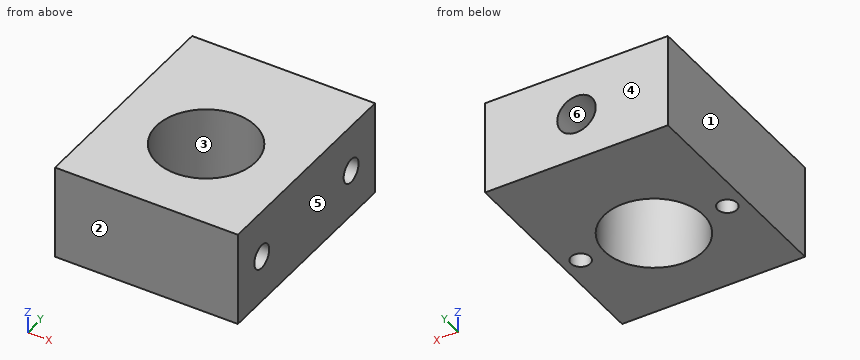
from build123d import *

# Parameters (mm, degrees)
F0_W     = 19
F0_H     = 23
F0_R     = 5.15
F1_DEPTH = 9.8
F3_D     = 2
F3_DEPTH = 5
F3_TIP   = 0.600860619
F5_D     = 4
F5_DEPTH = 5
F5_TIP   = 1.2017212381
F7_D     = 2.5
F7_DEPTH = 5
F7_TIP   = 0.7510757738


with BuildPart() as f1:
    # F0 (on Top) → F1 (new body)
    with BuildSketch(Plane.XY):
        with Locations((0, 1.5)):
            Rectangle(F0_W, F0_H)
        Circle(F0_R, mode=Mode.SUBTRACT)
    extrude(amount=F1_DEPTH)

    # F3
    with Locations(Plane(origin=(0, 0, 0), x_dir=(1, 0, 0), z_dir=(0, 0, -1))):
        with Locations((-7.62, 0), (7.62, 0)):
            Hole(F3_D / 2, depth=F3_DEPTH)
            with Locations((0, 0, -(F3_DEPTH + F3_TIP / 2))):  # 118° drill point
                Cone(0, F3_D / 2, F3_TIP, mode=Mode.SUBTRACT)

    # F5
    with Locations(Plane(origin=(0, 13, 0), x_dir=(-1, 0, 0), z_dir=(0, 1, 0))):
        with Locations((0, 4.9)):
            Hole(F5_D / 2, depth=F5_DEPTH)
            with Locations((0, 0, -(F5_DEPTH + F5_TIP / 2))):  # 118° drill point
                Cone(0, F5_D / 2, F5_TIP, mode=Mode.SUBTRACT)

    # F7
    with Locations(Plane.YZ.offset(9.5)):
        with Locations((-6, 4.9), (9, 4.9)):
            Hole(F7_D / 2, depth=F7_DEPTH)
            with Locations((0, 0, -(F7_DEPTH + F7_TIP / 2))):  # 118° drill point
                Cone(0, F7_D / 2, F7_TIP, mode=Mode.SUBTRACT)


solid = f1.part
Source: CAD feature listing. Evaluate the final solid. Frame: model axes, mm. Face numbers are marked on the shaded views. A direction names the side the tool comes from. Coordinates: 2 decimals unless noted, no trailing zeros. Loops run counter-clockwise (first coordinate to the right, second up) from the corner with the lowest first, then second, coordinate; pieces in that order, holes last. Notation, with made-up numbers: (46.5, 62) -> (69.5, 62) arc R12 ccw to (69.5, 69) -> close; hole circle Ø2 at (-27.5, 44). An arc over 180 degrees is marked (long way). Answer in a Markdown table with one row per item. Add a question column.
Q1. Section A-A on z = 1.5. Return the cut outline in (x, y), and give its area (3 significant figures).
Q2. Section C-C on x = 8. Give the number of separate pieces and of enclosed holes in the cut face, and give its area (3 significant figures).
Q3. Section B-B on y = 3.75. Return the cut outline in (x, z).
Q4. Reachability of the marked faces 5 and 6 from +Z, -Z, +X, -X, +Y, -Y: full face, straight path, thin tool, end or side. Return the list, or none.
Q5. Ray query, line 1 along Y through (x, z) = (7.65, 4.9); line 2 along Y through (x, z) = (6.5, 4.75); line 3 along Z through (x, y) = (0, 10.65). Return the intervals inside material, ascending.
Q6. Contact query for a flat-ended pin moving along its axis: pin 1 Ø2 at (y, z) = (9, 4.9) entering from +X. Output: stop coordinate, or through.
Q7. Pull-direction query (Y, two-part tool) for the marked faces 1, 2, 3 and 4; classes: pulls with the +Y half, pulls with the -Y half, needs draft (parallel to the pull), parting line crosses it, or undercut.
Computed values:
| question | item | result |
|---|---|---|
| 1 | outline | (-9.5, -10) -> (9.5, -10) -> (9.5, 13) -> (-9.5, 13) -> close; hole circle Ø2 at (-7.62, 0); hole circle Ø10.3 at (0, 0); hole circle Ø2 at (7.62, 0) |
| 1 | area | 347 mm^2 |
| 2 | separate pieces | 1 |
| 2 | enclosed holes | 2 |
| 2 | area | 206 mm^2 |
| 3 | outline | (-9.5, 0) -> (-3.53, 0) -> (-3.53, 9.8) -> (-9.5, 9.8) -> close; (3.53, 0) -> (9.5, 0) -> (9.5, 9.8) -> (3.53, 9.8) -> close |
| 4 | face 5 | +Z, -Z, +X, +Y, -Y |
| 4 | face 6 | +Y |
| 5 | line 1 | y = -10 to -7.25, -4.75 to -1, 1 to 7.75, 10.25 to 13 |
| 5 | line 2 | y = -10 to -7.24, -4.76 to 7.76, 10.24 to 13 |
| 5 | line 3 | z = 0 to 2.9, 6.9 to 9.8 |
| 6 | pin 1 | stops at x = 4.35 |
| 7 | face 1 | needs draft |
| 7 | face 2 | pulls with the -Y half |
| 7 | face 3 | undercut |
| 7 | face 4 | pulls with the +Y half |
